from build123d import *

# Parameters (mm, degrees)
SKETCH1_W            = 100
SKETCH1_H            = 77
BOSS_EXTRUDE1_DEPTH  = 3
BOSS_EXTRUDE2_DEPTH  = 20
SKETCH3_W            = 100
SKETCH3_H            = 3
BOSS_EXTRUDE3_DEPTH  = 3
SKETCH4_W            = 12
SKETCH4_H            = 23
CUT_EXTRUDE1_DEPTH   = 3
SKETCH5_R            = 1.5
CUT_EXTRUDE2_DEPTH   = 129.860389569
LPATTERN1_COUNT      = 2
LPATTERN1_PITCH      = 25
LPATTERN1_COUNT_DIR2 = 2
LPATTERN1_PITCH_DIR2 = 52
SKETCH6_R            = 1.4
CUT_EXTRUDE3_DEPTH   = 129.860389569
CUT_EXTRUDE4_REACH   = 130.86
SKETCH7_W            = 3
SKETCH7_H            = 8
CUT_EXTRUDE5_REACH   = 130.86
SKETCH9_R            = 1
FILLET1_R            = 3


with BuildPart() as part:
    # Sketch1 → Boss-Extrude1 (new body)
    with BuildSketch(Plane.XY):
        with Locations((-50, 38.5)):
            Rectangle(SKETCH1_W, SKETCH1_H)
    extrude(amount=BOSS_EXTRUDE1_DEPTH)

    # Sketch2 → Boss-Extrude2 (add)
    with BuildSketch(Plane.XY.offset(3)):
        Polygon((-100, 77), (-97, 77), (-3, 77), (0, 77), (0, 0), (-3, 0), (-3, 74), (-97, 74), (-97, 0), (-100, 0), align=None)
    extrude(amount=BOSS_EXTRUDE2_DEPTH)

    # Sketch3 → Boss-Extrude3 (add)
    with BuildSketch(Plane.XY.offset(23)):
        with Locations((-50, 75.5)):
            Rectangle(SKETCH3_W, SKETCH3_H)
    extrude(amount=BOSS_EXTRUDE3_DEPTH)

    # Sketch4 → Cut-Extrude1 (cut)
    with BuildSketch(Plane(origin=(0, 0, 0), x_dir=(-1, 0, 0), z_dir=(0, 0, -1))):
        with Locations((50, 56.5)):
            Rectangle(SKETCH4_W, SKETCH4_H)
    extrude(amount=-CUT_EXTRUDE1_DEPTH, mode=Mode.SUBTRACT)

    # Sketch5 → Cut-Extrude2 (cut, through all)
    with BuildSketch(Plane(origin=(0, 0, 0), x_dir=(-1, 0, 0), z_dir=(0, 0, -1))):
        with Locations((94, 10)):
            Circle(SKETCH5_R)
    cut_extrude2 = extrude(amount=-CUT_EXTRUDE2_DEPTH, mode=Mode.SUBTRACT)

    # LPattern1: Cut-Extrude2 2 × 2
    with Locations(*[(j * LPATTERN1_PITCH_DIR2, i * LPATTERN1_PITCH, 0) for i in range(LPATTERN1_COUNT) for j in range(LPATTERN1_COUNT_DIR2) if (i, j) != (0, 0)]):
        add(cut_extrude2, mode=Mode.SUBTRACT)

    # Sketch6 → Cut-Extrude3 (cut, through all)
    with BuildSketch(Plane(origin=(0, 0, 0), x_dir=(0, 0, -1), z_dir=(1, 0, 0))):
        with Locations(Location((-19, 4, 0), (0, 0, 90))):
            Circle(SKETCH6_R)
    cut_extrude3 = extrude(amount=-CUT_EXTRUDE3_DEPTH, mode=Mode.SUBTRACT)

    # Sketch7 → Cut-Extrude4 (cut, up to next)
    with BuildSketch(Plane.ZY.offset(100), mode=Mode.PRIVATE) as cut_extrude4_sk1:
        with Locations((5.5, 22.5)):
            Rectangle(SKETCH7_W, SKETCH7_H)
    cut_extrude4_tool1 = extrude(cut_extrude4_sk1.sketch, amount=-CUT_EXTRUDE4_REACH, mode=Mode.PRIVATE) & part.part
    add(cut_extrude4_tool1.solids().sort_by_distance((-100, 22.5, 5.5))[0], mode=Mode.SUBTRACT)

    # Sketch9 → Cut-Extrude5 (cut, up to next)
    with BuildSketch(Plane(origin=(0, 0, 0), x_dir=(-1, 0, 0), z_dir=(0, 0, -1)), mode=Mode.PRIVATE) as cut_extrude5_sk1:
        with Locations((50, 71)):
            Circle(SKETCH9_R)
    cut_extrude5_tool1 = extrude(cut_extrude5_sk1.sketch, amount=-CUT_EXTRUDE5_REACH, mode=Mode.PRIVATE) & part.part
    cut_extrude5 = cut_extrude5_tool1.solids().sort_by_distance((-50, 71, 0))[0]
    add(cut_extrude5, mode=Mode.SUBTRACT)

    # Mirror1: Cut-Extrude5 across plane
    add(cut_extrude5.mirror(Plane(origin=(0, 56.5, 0), x_dir=(0, 0, 1), z_dir=(0, -1, 0))), mode=Mode.SUBTRACT)

    # Mirror2: Cut-Extrude3 across plane
    add(cut_extrude3.mirror(Plane(origin=(0, 37, 0), x_dir=(0, 0, 1), z_dir=(0, -1, 0))), mode=Mode.SUBTRACT)

    # Fillet1
    fillet1_edges = [part.edges().sort_by_distance(p)[0] for p in [
        (0, 77, 13),
        (-100, 77, 13),
    ]]
    fillet(fillet1_edges, radius=FILLET1_R - 0.0001)  # a hair under: the kernel refuses the full size


solid = part.part
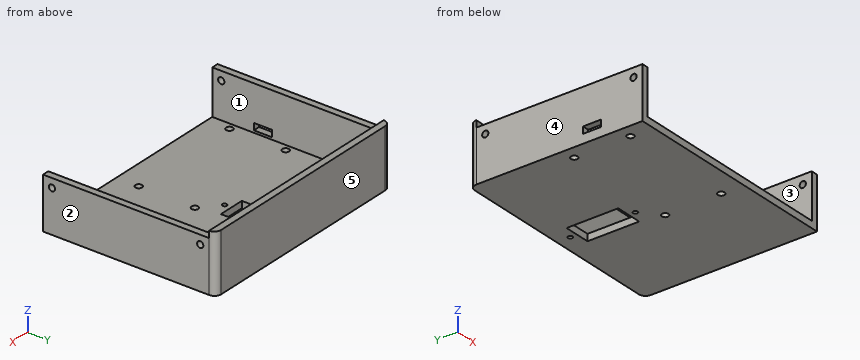
The listing builds one solid part. Answer for the finished solid, in the listing's coordinates (mm). Face numbers are marked on the shaded views. A direction names the side the tool comes from. Give positions to 0.01 mm unless a question says otherwise; leave off trailing zeros. Write each loop counter-clockwise with the first axis right and the second up, starting at its lowest first coordinate (ties: lowest second). Pieces come first, ordered by that corner, then holes. Notation, with made-up numbers: (16.25, -39.5) - (59.25, -39.5) arc R24 ccw to (59.25, -16.5) - close; hole circle Ø7 at (7, -27). An arc over 180 degrees is marked (long way). One line per question, with ' | ' between items. Start each with the question number.
1. Section D-D, the plane x = -94 is taken. Determine the outline of the cut face in (y, z).
2. Determine the mould class of the marked faces 3, 4 and 5 for opening direction X: +X half, -X half, draft (parallel to the pull), parting line (faces both ways), or undercut.
3. Section B-B, the plane x = -46.5 is taken. Determine the outline of the cut face in (y, z), then the cut area to 3 significant figures.
4. For the marked faces 1 and 2, determine the directions among +Z, -Z, +X, -X, +Y, -Y from which every point of the face is accessible in a straight line to the end or side of a thin tool.
5. Section C-C, the plane y = 10 is taken. Determine the outline of the cut face in (x, z), then the cut area to 3 significant figures.
6. Given P1, Ø0.9, axis at x = -99, z = 6, coming from the -Y side; P2, Ø2.5, axis at x = -50, y = 42, coming from the +Z side; P3, Ø2.5, axis at x = -42, y = 35, coming from the -Z side; P4, Ø1, axis at x = -16.5, z = 20.5, coming from the -Y side, each flat-ended and moving along its own axis, determine where each tip first touches the part or whether it passes through.
7. Straight lines are drawn through the part: line 1 (X direction, y = 31, z = 3.75); line 2 (Y direction, x = -50, z = 2.1); line 3 (Z direction, x = -17, y = 20). For each, find the intervals that lie inside material, in ascending order.
8. Section A-A, the plane y = 60.5 is taken. Determine the outline of the cut face in (x, z).
Result:
1) outline: (0, 0) - (8.5, 0) - (8.5, 3) - (0, 3) - close; (11.5, 0) - (33.5, 0) - (33.5, 3) - (11.5, 3) - close; (36.5, 0) - (77, 0) - (77, 26) - (74, 26) - (74, 3) - (36.5, 3) - close
2) face 3: undercut | face 4: -X half | face 5: draft
3) outline: (0, 0) - (45, 0) - (45, 3) - (0, 3) - close; (68, 0) - (77, 0) - (77, 26) - (74, 26) - (74, 3) - (68, 3) - close | area: 231 mm2
4) face 1: +Z, -Y | face 2: +Z, -Z, +X, +Y, -Y
5) outline: (-100, 0) - (-95.5, 0) - (-95.5, 3) - (-97, 3) - (-97, 23) - (-100, 23) - close; (-92.5, 0) - (-43.5, 0) - (-43.5, 3) - (-92.5, 3) - close; (-40.5, 0) - (0, 0) - (0, 23) - (-3, 23) - (-3, 3) - (-40.5, 3) - close | area: 402 mm2
6) P1: stops at y = 0 | P2: stops at z = 3 | P3: passes through | P4: stops at y = 74
7) line 1: x = -100 to -97, -3 to 0 | line 2: y = 0 to 41, 43 to 45, 68 to 70, 72 to 77 | line 3: z = 0 to 3
8) outline: (-100, 0) - (-56, 0) - (-56, 3) - (-97, 3) - (-97, 23) - (-100, 23) - close; (-44, 0) - (0, 0) - (0, 23) - (-3, 23) - (-3, 3) - (-44, 3) - close
